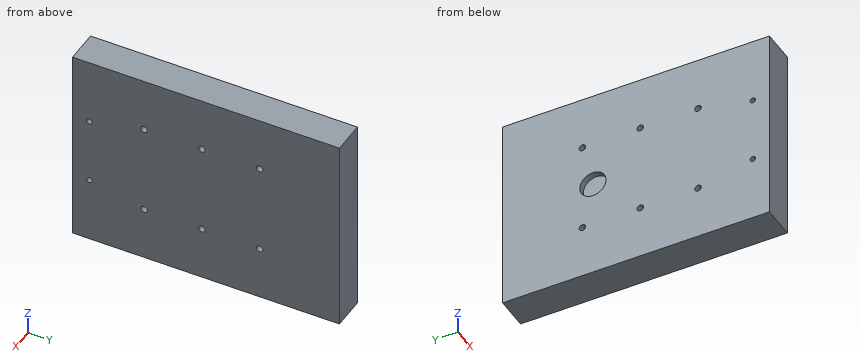
from build123d import *

# Parameters (mm, degrees)
SKETCH2_W                          = 76.2
SKETCH2_H                          = 101.6
BOSS_EXTRUDE2_DEPTH                = 12.7
F_2_5MM_DOWEL_HOLE1_D              = 2.5
SKETCH5_R                          = 5
CUT_EXTRUDE1_DEPTH                 = 2.5
TAP_DRILL_FOR_M2_5X0_45_TAP1_D     = 2.05
TAP_DRILL_FOR_M2_5X0_45_TAP1_DEPTH = 12.7
TAP_DRILL_FOR_M2_5X0_45_TAP1_TIP   = 0.615882135


with BuildPart() as part:
    # Sketch2 → Boss-Extrude2 (new body)
    with BuildSketch(Plane(origin=(0, 0, 0), x_dir=(0, 0, -1), z_dir=(1, 0, 0))):
        with Locations((0, 50.8)):
            Rectangle(SKETCH2_W, SKETCH2_H)
    extrude(amount=BOSS_EXTRUDE2_DEPTH)

    # Ø2.5mm Dowel Hole1 (through all)
    with Locations(Plane.ZY):
        with Locations((-17.3, 71.2), (-17.3, 49.2), (-17.3, 27.2)):
            f_2_5mm_dowel_hole1 = Hole(F_2_5MM_DOWEL_HOLE1_D / 2)

    # Mirror1: Ø2.5mm Dowel Hole1 across plane
    add(f_2_5mm_dowel_hole1.mirror(Plane.XY), mode=Mode.SUBTRACT)

    # Sketch5 → Cut-Extrude1 (cut)
    with BuildSketch(Plane.ZY):
        with Locations((0, 67.2)):
            Circle(SKETCH5_R)
    extrude(amount=-CUT_EXTRUDE1_DEPTH, mode=Mode.SUBTRACT)

    # Tap Drill for M2.5x0.45 Tap1
    with Locations(Plane(origin=(12.7, 0, 0), x_dir=(0, 0, -1), z_dir=(1, 0, 0))):
        with Locations((-12.7, 6.35), (12.7, 6.35)):
            Hole(TAP_DRILL_FOR_M2_5X0_45_TAP1_D / 2, depth=TAP_DRILL_FOR_M2_5X0_45_TAP1_DEPTH)
            with Locations((0, 0, -(TAP_DRILL_FOR_M2_5X0_45_TAP1_DEPTH + TAP_DRILL_FOR_M2_5X0_45_TAP1_TIP / 2))):  # 118° drill point
                Cone(0, TAP_DRILL_FOR_M2_5X0_45_TAP1_D / 2, TAP_DRILL_FOR_M2_5X0_45_TAP1_TIP, mode=Mode.SUBTRACT)


solid = part.part
Input: part model. Units: mm. Frame: model coordinates. Coordinates: 2 decimals unless noted, no trailing zeros. Loops run counter-clockwise (first coordinate to the right, second up) from the corner with the lowest first, then second, coordinate; pieces in that order, holes last.
Q1. Cut plane D-D (y = 67.2). Output: boundary loops of the cut face in (x, z), then the cut area to 3 significant figures.
Q2. Cut plane C-C (z = -12.7). Output: boundary loops of the cut face in (x, y) (3 decimals), then the cut area to 3 significant figures.
Q3. Contact query for flat-ended pins moving along their axis: pin 1 (2.5 mm diameter, centred on y = 6.35, z = -12.7, fed in from -X); pin 2 (8 mm diameter, centred on y = 68, z = -0.5, fed in from -X). Output: stop coordinate, or through.
Q4. Cut plane A-A (y = 49.2). Output: boundary loops of the cut face in (x, z), then the cut area to 3 significant figures.
Q5. Cut plane B-B (z = 17.3). Output: boundary loops of the cut face in (x, y), then the cut area to 3 significant figures.
Q6. Material intervals for line 1 (Y direction, x = 5.5, z = -17.3); line 2 (Z direction, x = 8.75, y = 6.35) (3 decimals); line 3 (Z direction, x = 8.75, y = 27), sorted ascending.
Working result:
1. outline: (0, -38.1) - (12.7, -38.1) - (12.7, 38.1) - (0, 38.1) - (0, 5) - (2.5, 5) - (2.5, -5) - (0, -5) - close
1. area: 943 mm2
2. outline: (0, 0) - (12.7, 0) - (12.7, 5.325) - (0, 5.325) - close; (0, 7.375) - (12.7, 7.375) - (12.7, 101.6) - (0, 101.6) - close
2. area: 1,260 mm2
3. pin 1: stops at x = 0
3. pin 2: stops at x = 2.5
4. outline: (0, -38.1) - (12.7, -38.1) - (12.7, -18.55) - (0, -18.55) - close; (0, -16.05) - (12.7, -16.05) - (12.7, 16.05) - (0, 16.05) - close; (0, 18.55) - (12.7, 18.55) - (12.7, 38.1) - (0, 38.1) - close
4. area: 904 mm2
5. outline: (0, 0) - (12.7, 0) - (12.7, 25.95) - (0, 25.95) - close; (0, 28.45) - (12.7, 28.45) - (12.7, 47.95) - (0, 47.95) - close; (0, 50.45) - (12.7, 50.45) - (12.7, 69.95) - (0, 69.95) - close; (0, 72.45) - (12.7, 72.45) - (12.7, 101.6) - (0, 101.6) - close
5. area: 1,200 mm2
6. line 1: y = 0 to 25.95, 28.45 to 47.95, 50.45 to 69.95, 72.45 to 101.6
6. line 2: z = -38.1 to -13.725, -11.675 to 11.675, 13.725 to 38.1
6. line 3: z = -38.1 to -18.53, -16.07 to 16.07, 18.53 to 38.1
